from build123d import *

# Parameters (mm, degrees)
BOSS_EXTRUDE1_DEPTH = 2
BOSS_EXTRUDE2_DEPTH = 1.5
BOSS_EXTRUDE3_DEPTH = 2.3
SKETCH6_W           = 4
SKETCH6_H           = 4.5
CUT_EXTRUDE1_DEPTH  = 2
SKETCH7_R           = 3
CUT_EXTRUDE2_DEPTH  = 3.3
SKETCH8_W           = 13.393145751
SKETCH8_H           = 2
SKETCH8_W_2         = 10.05
SKETCH8_H_2         = 1.5
BOSS_EXTRUDE4_DEPTH = 1.2
SKETCH9_R           = 2.5
BOSS_EXTRUDE5_DEPTH = 1.2
SKETCH10_R          = 0.95
CUT_EXTRUDE3_DEPTH  = 8.2
SKETCH11_R          = 2
CUT_EXTRUDE4_DEPTH  = 2.2
FILLET1_R           = 1.5
FILLET2_R           = 1
FILLET3_R           = 2
SKETCH13_W          = 3
SKETCH13_H          = 8
BOSS_EXTRUDE6_DEPTH = 12
SKETCH14_R          = 1.5
CUT_EXTRUDE5_DEPTH  = 12


with BuildPart() as part:
    # Sketch2 → Boss-Extrude1 (new body)
    with BuildSketch(Plane.XY):
        with BuildLine():
            Line((4.95, 7.456854249), (24.343145751, 7.456854249))
            Line((24.343145751, 7.456854249), (24.343145751, 5.656854249))
            ThreePointArc((24.343145751, 5.656854249), (22.60896374, 3.061467459), (22, 0))
            Line((22, 0), (21, -2.543145751))
            Line((21, -2.543145751), (21, -7.043145751))
            Line((21, -7.043145751), (8.499747468, -7.043145751))
            Line((8.499747468, -7.043145751), (4.95, -7.043145751))
            Line((4.95, -7.043145751), (4.95, 7.456854249))
        make_face()
    extrude(amount=BOSS_EXTRUDE1_DEPTH)

    # Sketch3 → Boss-Extrude2 (add)
    with BuildSketch(Plane.XY.offset(2)):
        with BuildLine():
            Line((24.343145751, 7.456854249), (24.343145751, 5.656854249))
            ThreePointArc((24.343145751, 5.656854249), (22.60896374, 3.061467459), (22, 0))
            Line((22, 0), (21, -2.543145751))
            Line((21, -2.543145751), (21, -7.043145751))
            Line((21, -7.043145751), (21, -8.543145751))
            Line((21, -8.543145751), (4.95, -8.543145751))
            Line((4.95, -8.543145751), (4.95, 8.956854249))
            Line((4.95, 8.956854249), (24.343145751, 8.956854249))
            Line((24.343145751, 8.956854249), (24.343145751, 7.456854249))
        make_face()
    extrude(amount=BOSS_EXTRUDE2_DEPTH)

    # Sketch5 → Boss-Extrude3 (add)
    with BuildSketch(Plane.XY.offset(3.5)):
        with BuildLine():
            Line((4.95, -8.543145751), (21, -8.543145751))
            Line((21, -8.543145751), (21, -5.656854249))
            Line((21, -5.656854249), (30.003145751, -5.656854249))
            ThreePointArc((30.003145751, -5.656854249), (35.66, 0), (30.003145751, 5.656854249))
            Line((30.003145751, 5.656854249), (24.343145751, 5.656854249))
            Line((24.343145751, 5.656854249), (24.343145751, 7.5))
            Line((24.343145751, 7.5), (24.343145751, 8.956854249))
            Line((24.343145751, 8.956854249), (4.95, 8.956854249))
            Line((4.95, 8.956854249), (4.95, -8.543145751))
        make_face()
    extrude(amount=BOSS_EXTRUDE3_DEPTH)

    # Sketch6 → Cut-Extrude1 (cut)
    with BuildSketch(Plane.XY.offset(5.8)):
        with Locations((6.95, 5.206854249)):
            Rectangle(SKETCH6_W, SKETCH6_H)
        with Locations((6.95, -4.793145751)):
            Rectangle(SKETCH6_W, SKETCH6_H)
    extrude(amount=-CUT_EXTRUDE1_DEPTH, mode=Mode.SUBTRACT)

    # Sketch7 → Cut-Extrude2 (cut)
    with BuildSketch(Plane.XY.offset(5.8)):
        with Locations((30.003145751, 0)):
            Circle(SKETCH7_R)
    extrude(amount=-CUT_EXTRUDE2_DEPTH, mode=Mode.SUBTRACT)

    # Sketch8 → Boss-Extrude4 (add)
    with BuildSketch(Plane.XY.offset(5.8)):
        with Locations((17.646572876, 7.956854249)):
            Rectangle(SKETCH8_W, SKETCH8_H)
        with Locations((15.975, -7.793145751)):
            Rectangle(SKETCH8_W_2, SKETCH8_H_2)
        with BuildLine():
            Line((10.95, -4.172114809), (21.343145751, -4.172114809))
            ThreePointArc((21.343145751, -4.172114809), (22.343145751, -3.172114809), (21.343145751, -2.172114809))
            Line((21.343145751, -2.172114809), (10.95, -2.172114809))
            Line((10.95, -2.172114809), (10.95, -4.172114809))
        make_face()
        with BuildLine():
            Line((21.343145751, 4.180295218), (10.95, 4.180295218))
            Line((10.95, 4.180295218), (10.95, 2.180295218))
            Line((10.95, 2.180295218), (21.343145751, 2.180295218))
            ThreePointArc((21.343145751, 2.180295218), (22.343145751, 3.180295218), (21.343145751, 4.180295218))
        make_face()
    extrude(amount=BOSS_EXTRUDE4_DEPTH)

    # Sketch9 → Boss-Extrude5 (add)
    with BuildSketch(Plane.XY.offset(5.8)):
        with Locations((18.5, 0)):
            Circle(SKETCH9_R)
        with Locations((12, 0)):
            Circle(SKETCH9_R)
    extrude(amount=BOSS_EXTRUDE5_DEPTH)

    # Sketch10 → Cut-Extrude3 (cut)
    with BuildSketch(Plane.XY.offset(7)):
        with Locations((18.5, 0)):
            Circle(SKETCH10_R)
        with Locations((12, 0)):
            Circle(SKETCH10_R)
    extrude(amount=-CUT_EXTRUDE3_DEPTH, mode=Mode.SUBTRACT)

    # Sketch11 → Cut-Extrude4 (cut)
    with BuildSketch(Plane(origin=(0, 0, 0), x_dir=(-1, 0, 0), z_dir=(0, 0, -1))):
        with Locations((-12, 0)):
            Circle(SKETCH11_R)
        with Locations((-18.5, 0)):
            Circle(SKETCH11_R)
    extrude(amount=-CUT_EXTRUDE4_DEPTH, mode=Mode.SUBTRACT)

    # Fillet1
    fillet1_edges = [part.edges().sort_by_distance(p)[0] for p in [
        (14.646572875, 8.956854249, 2),
        (12.975, -8.543145751, 2),
    ]]
    fillet(fillet1_edges, radius=FILLET1_R - 0.0001)  # a hair under: the kernel refuses the full size

    # Fillet2
    fillet2_edges = [part.edges().sort_by_distance(p)[0] for p in [
        (12.975, -7.043145751, 0),
        (14.646572875, 7.456854249, 0),
    ]]
    fillet(fillet2_edges, radius=FILLET2_R)

    # Fillet3
    fillet3_edges = [part.edges().sort_by_distance(p)[0] for p in [
        (8.95, -4.793145751, 5.8),
        (8.95, 5.206854249, 5.8),
    ]]
    fillet(fillet3_edges, radius=FILLET3_R - 0.0001)  # a hair under: the kernel refuses the full size

    # Sketch13 → Boss-Extrude6 (add)
    with BuildSketch(Plane.ZY.offset(-4.95)):
        with Locations((1.5, 0)):
            Rectangle(SKETCH13_W, SKETCH13_H)
    extrude(amount=BOSS_EXTRUDE6_DEPTH)

    # Sketch14 → Cut-Extrude5 (cut)
    with BuildSketch(Plane(origin=(0, 0, 0), x_dir=(-1, 0, 0), z_dir=(0, 0, -1))):
        with Locations((-1.95, 0)):
            Circle(SKETCH14_R)
        with Locations((4.05, 0)):
            Circle(SKETCH14_R)
    extrude(amount=-CUT_EXTRUDE5_DEPTH, mode=Mode.SUBTRACT)


solid = part.part
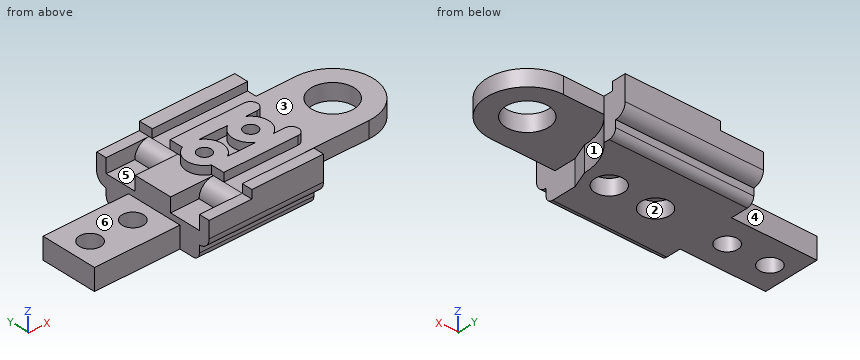
Input: part model. Units: mm. Frame: model coordinates. Face numbers are marked on the shaded views. A direction names the side the tool comes from. Coordinates: 2 decimals unless noted, no trailing zeros. Write each loop counter-clockwise with the first axis right and the second up, starting at its lowest first coordinate (ties: lowest second). Pieces come first, ordered by that corner, then holes. Notation, with made-up numbers: M -15,29.5 L 35,29.5 A26 ccw 35,45.5 Z; hole C 30.5,38 d9. An arc over 180 degrees is marked long. Answer as a JSON object with one key per item and string values. Group by question number.
(1) Mould query, pull axis Y, two halves, no side actions, for the marked faces 4, 5 and 6. Classes: pulls with the +Y half, pulls with the -Y half, needs draft (parallel to the pull), parting line crosses it, or undercut.
(2) Ray query, line 1 along Y through (x, z) = (12, 1.15); line 2 along Y through (x, z) = (12, 4.2); line 3 along X through (y, z) = (0.25, 4.25). Return the intervals inside material, ascending. Write a range as [from, to].
(3) Section A-A on z = 6.25. Output: boundary loops of the cut face in (x, y).
(4) Section B-B on x = 1.95. Output: boundary loops of the cut face in (y, z), plus the area to 3 significant figures.
(5) Section D-D on z = 0.5. Output: boundary loops of the cut face in (x, y).
(6) Contact query for flat-ended pins moving along their axis: P1, Ø3, axis at x = 12, y = 0, coming from the +Z side; P2, Ø3.5, axis at x = -4.05, y = 0, coming from the +Z side; P3, Ø1.2, axis at x = 26, z = 4.5, coming from the -Y side; P4, Ø2.5, axis at x = 1.95, y = 0, coming from the -Z side (3 decimals). Output: stop coordinate, or through.
(7) Set-up query: the marked faces 1, 2 and 3. Return all of +Z, -Z, +X, -X, +Y, -Y with unobstructed straight access to the full face (end or side cutting, diameter ignored); none if empty.
Result set:
{
 "1": {"face 4": "pulls with the +Y half", "face 5": "undercut", "face 6": "needs draft"},
 "2": {"line 1": "y = [-7.04, -2], [2, 7.46]", "line 2": "y = [-8.54, -0.95], [0.95, 8.96]", "line 3": "x = [4.95, 11.08], [12.92, 17.58], [19.42, 27.01], [32.99, 35.65]"},
 "3": {"outline": "M 10.95,-8.54 L 21,-8.54 L 21,-7.04 L 10.95,-7.04 Z; M 10.95,-4.17 L 21.34,-4.17 A1 ccw 21.34,-2.17 L 19.74,-2.17 A2.5 ccw 19.72,2.18 L 21.34,2.18 A1 ccw 21.34,4.18 L 10.95,4.18 L 10.95,2.27 A2.5 ccw 10.95,-2.27 Z; M 10.95,6.96 L 24.34,6.96 L 24.34,8.96 L 10.95,8.96 Z; hole C 12,0 d1.9; hole M 13.22,2.18 A2.5 cw 13.24,-2.17 L 17.26,-2.17 A2.5 cw 17.28,2.18 Z; hole C 18.5,0 d1.9"},
 "4": {"outline": "M -4,0 L -1.5,0 L -1.5,3 L -4,3 Z; M 1.5,0 L 4,0 L 4,3 L 1.5,3 Z", "area": "15.0 mm2"},
 "5": {"outline": "M -7.05,-4 L 4.95,-4 L 4.95,-6.91 L 21,-6.91 L 21,-2.54 L 22,0 A8 cw 24.34,5.66 L 24.34,7.32 L 4.95,7.32 L 4.95,4 L -7.05,4 Z; hole C -4.05,0 d3; hole C 1.95,0 d3; hole C 12,0 d4; hole C 18.5,0 d4"},
 "6": {"P1": "stops at z = 7", "P2": "stops at z = 3", "P3": "stops at y = -5.66", "P4": "passes through"},
 "7": {"face 1": "-Z, +X, -Y", "face 2": "-Z", "face 3": "+Z"}
}
